For this review, take the finished solid that the model builds, in its own axes (mm). A direction names the side the tool comes from. Coordinates: 2 decimals unless noted, no trailing zeros. Loops run counter-clockwise (first coordinate to the right, second up) from the corner with the lowest first, then second, coordinate; pieces in that order, holes last.
1. Take a section at A-A, the plane z = -85. State the section outline as (x, y) points, then the cut area to 4 significant figures.
2. Mouldability with a two-part tool opening along X and no side actions: class faces 1 (the face through (12.5, 3.5, -14.9)), 2 (the face through (145.95, 3.45, -50.9)), 3 (the face through (186.39, 3.55, -96.58)), 4 (the face through (88, 3, 0)) as pulls with the +X half, pulls with the -X half, needs draft (parallel to the pull), parting line crosses it, or undercut.
3. To check wall thickness, follow probe 1 along Z at (x, y) = (32, 3.5); probe 2 along X at (y, z) = (5.5, -50); probe 3 along Z at (x, y) = (13, 0.75). State the ranges of each line that lie inside material, in increasing order.
4. Take a section at C-C, the plane y = 2.25. Count the separate pieces of the cut face and the enclosed holes in it, then the cut area to 3 significant figures.
5. Take a section at B-B, the plane x = 150. State the section outline as (y, z) points, then the cut area to 3 significant figures.
6. Machinability: for faces 5 (the face through (0, 3, -49)), 6 (the face through (30, 3, -17.5)), which of the approach directions +Z, -Z, +X, -X, +Y, -Y give a long, thin tool a straight path to every point of the face, cutting with its end or side? Answer none if there is none.
7. Take a section at D-D, the plane z = -50. State the section outline as (x, y) points, then the cut area to 3 significant figures.
```python
from build123d import *

# Parameters (mm, degrees)
SKETCH1_W           = 190
SKETCH1_H           = 100
SKETCH1_R           = 4.15
SKETCH1_R_2         = 4.1
SKETCH1_R_3         = 2.6
BOSS_EXTRUDE1_DEPTH = 7
FILLET3_R           = 12


with BuildPart() as part:
    # Sketch1 → Boss-Extrude1 (new body)
    with BuildSketch(Plane(origin=(0, 0, 0), x_dir=(1, 0, 0), z_dir=(0, 1, 0))):
        with Locations((95, 50)):
            Rectangle(SKETCH1_W, SKETCH1_H)
        with Locations(Location((150, 50, 0), (0, 0, 270))):
            Circle(SKETCH1_R, mode=Mode.SUBTRACT)
        with Locations(Location((150, 74, 0), (0, 0, 270))):
            Circle(SKETCH1_R_2, mode=Mode.SUBTRACT)
        with Locations(Location((131.75, 50, 0), (0, 0, 270))):
            Circle(SKETCH1_R_3, mode=Mode.SUBTRACT)
        with Locations(Location((168.25, 50, 0), (0, 0, 270))):
            Circle(SKETCH1_R_3, mode=Mode.SUBTRACT)
        with Locations(Location((150, 26, 0), (0, 0, 270))):
            Circle(SKETCH1_R_2, mode=Mode.SUBTRACT)
        with BuildLine():
            Line((160, 12.5), (180, 12.5))
            ThreePointArc((180, 12.5), (182.5, 10), (180, 7.5))
            Line((180, 7.5), (160, 7.5))
            ThreePointArc((160, 7.5), (157.5, 10), (160, 12.5))
        make_face(mode=Mode.SUBTRACT)
        with BuildLine():
            Line((160, 87.5), (180, 87.5))
            ThreePointArc((180, 87.5), (182.5, 90), (180, 92.5))
            Line((180, 92.5), (160, 92.5))
            ThreePointArc((160, 92.5), (157.5, 90), (160, 87.5))
        make_face(mode=Mode.SUBTRACT)
        with BuildLine():
            Line((15, 87.5), (45, 87.5))
            ThreePointArc((45, 87.5), (47.5, 85), (45, 82.5))
            Line((45, 82.5), (15, 82.5))
            ThreePointArc((15, 82.5), (12.5, 85), (15, 87.5))
        make_face(mode=Mode.SUBTRACT)
        with BuildLine():
            Line((15, 52.5), (45, 52.5))
            ThreePointArc((45, 52.5), (47.5, 50), (45, 47.5))
            Line((45, 47.5), (15, 47.5))
            ThreePointArc((15, 47.5), (12.5, 50), (15, 52.5))
        make_face(mode=Mode.SUBTRACT)
        with BuildLine():
            Line((15, 17.5), (45, 17.5))
            ThreePointArc((45, 17.5), (47.5, 15), (45, 12.5))
            Line((45, 12.5), (15, 12.5))
            ThreePointArc((15, 12.5), (12.5, 15), (15, 17.5))
        make_face(mode=Mode.SUBTRACT)
    extrude(amount=BOSS_EXTRUDE1_DEPTH)

    # Fillet3
    fillet3_edges = [part.edges().sort_by_distance(p)[0] for p in [
        (190, 3.5, -100),
        (190, 3.5, 0),
    ]]
    fillet(fillet3_edges, radius=FILLET3_R)


solid = part.part
```
Results list:
1. outline: (0, 0) - (12.5, 0) - (12.5, 7) - (0, 7) - close; (47.5, 0) - (190, 0) - (190, 7) - (47.5, 7) - close
1. area: 1,085 mm2
2. face 1: undercut
2. face 2: undercut
2. face 3: pulls with the +X half
2. face 4: needs draft
3. probe 1: z = -100 to -87.5, -82.5 to -52.5, -47.5 to -17.5, -12.5 to 0
3. probe 2: x = 0 to 12.5, 47.5 to 129.15, 134.35 to 145.85, 154.15 to 165.65, 170.85 to 190
3. probe 3: z = -100 to -86.5, -83.5 to -51.5, -48.5 to -16.5, -13.5 to 0
4. separate pieces: 1
4. enclosed holes: 10
4. area: 18,000 mm2
5. outline: (0, -100) - (7, -100) - (7, -78.1) - (0, -78.1) - close; (0, -69.9) - (7, -69.9) - (7, -54.15) - (0, -54.15) - close; (0, -45.85) - (7, -45.85) - (7, -30.1) - (0, -30.1) - close; (0, -21.9) - (7, -21.9) - (7, 0) - (0, 0) - close
5. area: 527 mm2
6. face 5: +Z, -Z, -X, +Y, -Y
6. face 6: +Y, -Y
7. outline: (0, 0) - (12.5, 0) - (12.5, 7) - (0, 7) - close; (47.5, 0) - (129.15, 0) - (129.15, 7) - (47.5, 7) - close; (134.35, 0) - (145.85, 0) - (145.85, 7) - (134.35, 7) - close; (154.15, 0) - (165.65, 0) - (165.65, 7) - (154.15, 7) - close; (170.85, 0) - (190, 0) - (190, 7) - (170.85, 7) - close
7. area: 954 mm2
